```python
from build123d import *

# Parameters (mm, degrees)
ENL_V_MAT_EXTRU_1_DEPTH = 1


with BuildPart() as part:
    # Esquisse1 → Révolution1 (revolve)
    with BuildSketch(Plane.XY, mode=Mode.PRIVATE) as r_volution1_sk:
        Polygon((10, 3), (-10, 3), (-10, 1.5), (-15, 1.5), (-15, 2.75), (-15.5, 2.75), (-16.5, 1.75), (-16.5, 0), (16.5, 0), (16.5, 1.75), (15.5, 2.75), (15, 2.75), (15, 1.5), (10, 1.5), align=None)
    revolve(r_volution1_sk.sketch.rotate(Axis((0, 0, 0), (-1, 0, 0)), 90), axis=Axis((0, 0, 0), (-1, 0, 0)))

    # Esquisse2 → Enlèv. mat.-Extru.1 (cut)
    with BuildSketch(Plane(origin=(16.5, 0, 0), x_dir=(0, 0, -1), z_dir=(1, 0, 0))):
        Polygon((0.577350269, 1), (-0.577350269, 1), (-1.154700538, 0), (-0.577350269, -1), (0.577350269, -1), (1.154700538, 0), align=None)
    enl_v_mat_extru_1 = extrude(amount=-ENL_V_MAT_EXTRU_1_DEPTH, mode=Mode.SUBTRACT)

    # Symétrie1: Enlèv. mat.-Extru.1 across plane
    add(enl_v_mat_extru_1.mirror(Plane(origin=(0, 0, 0), x_dir=(0, 0, 1), z_dir=(1, 0, 0))), mode=Mode.SUBTRACT)


solid = part.part
```
Verification items for the finished model (mm, model axes). A direction names the side the tool comes from. Give positions to 0.01 mm unless a question says otherwise; leave off trailing zeros. Loops run counter-clockwise (first coordinate to the right, second up) from the corner with the lowest first, then second, coordinate; pieces in that order, holes last.
1. Set-up check for faces 1 (the flat face through (-15, 1.2, 1.2)), 2 (the flat face through (-16, -1, 0)), 3 (the flat face through (16, -1, 0)): record each of +Z, -Z, +X, -X, +Y, -Y from which the full face is reachable in a straight line by a thin tool's end or side.
2. Section check B-B, the plane x = -13. Enter the section's corners in (y, z).
3. Section check C-C, the plane y = 2.35. Count the separate pieces of the cut face and the enclosed holes in it, then the cut area to 3 significant figures.
4. Go/stop test with flat-tipped pins: pin 1 Ø1.6 at (y, z) = (0, 0) entering from +X; pin 2 Ø0.5 at (x, z) = (-16, 0.5) entering from +Y; pin 3 Ø0.5 at (x, z) = (-16, 0.5) entering from -Y. Record where each tip stops, or that it passes through.
5. Thickness scan on line 1 (X direction, y = -1.3, z = 0.9); line 2 (X direction, y = 0.4, z = -2.5); line 3 (Z direction, x = -14.5, y = -0.1). Record the ranges inside material, lowest first.
6. Mould release check, pull along X, two halves, no side actions. Record for faces 4 (the flat face through (-16.5, 1, -1)), 5 (the flat face through (-16.01, 0.49, -0.87)), 6 (the flat face through (-10, 1.3, -1.3)): released by +X, released by -X, zero draft, split by the parting line, or undercut.
Geometry says:
1. face 1: none
1. face 2: -X
1. face 3: +X
2. outline: circle Ø3 at (0, 0)
3. separate pieces: 3
3. enclosed holes: 0
3. area: 78.9 mm2
4. pin 1: stops at x = 15.5
4. pin 2: stops at y = 2.45
4. pin 3: stops at y = -2.45
5. line 1: x = -16.5 to -15, -10 to 10, 15 to 16.5
5. line 2: x = -15.72 to -15, -10 to 10, 15 to 15.72
5. line 3: z = -1.5 to 1.5
6. face 4: released by -X
6. face 5: zero draft
6. face 6: undercut
